Geometry check sheet. Reference: the model listing, model coordinates, mm. Give positions to 0.01 mm unless a question says otherwise; leave off trailing zeros. Write each loop counter-clockwise with the first axis right and the second up, starting at its lowest first coordinate (ties: lowest second). Pieces come first, ordered by that corner, then holes. Notation, with made-up numbers: (-17, -5) - (18, -5) arc R19 cw to (18, 18) - close; hole circle Ø4 at (36, 54). An arc over 180 degrees is marked (long way). Use a Markdown table: item, result.
```python
from build123d import *

# Parameters (mm, degrees)
SKETCH_1_W          = 376.5
SKETCH_1_H          = 280
EXTRUDE_1_DEPTH     = 5
SKETCH_2_R          = 26.25
CUT_EXTRUDE_1_DEPTH = 5
SKETCH_3_R          = 3
EXTRUDE_2_DEPTH     = 5
EXTRUDE_START       = 5
SKETCH_4_R          = 3
EXTRUDE_3_DEPTH     = 5


with BuildPart() as part:
    # 草图1 → 凸台-拉伸1 (new body)
    with BuildSketch(Plane.XY):
        with Locations((188.25, 140)):
            Rectangle(SKETCH_1_W, SKETCH_1_H)
    extrude(amount=EXTRUDE_1_DEPTH)

    # 草图2 → 切除-拉伸1 (cut)
    with BuildSketch(Plane.XY.offset(5)):
        with Locations(Location((84.25, 203.497422612, 0), (0, 0, 180))):
            Circle(SKETCH_2_R)
        with Locations(Location((188.25, 228.989690448, 0), (0, 0, 180))):
            Circle(SKETCH_2_R)
        with Locations(Location((160.25, 180.492267836, 0), (0, 0, 180))):
            Circle(SKETCH_2_R)
        with Locations(Location((216.25, 180.492267836, 0), (0, 0, 180))):
            Circle(SKETCH_2_R)
        with Locations(Location((244.25, 131.994845224, 0), (0, 0, 180))):
            Circle(SKETCH_2_R)
        with Locations(Location((132.25, 131.994845224, 0), (0, 0, 180))):
            Circle(SKETCH_2_R)
        with Locations(Location((188.25, 131.994845224, 0), (0, 0, 180))):
            Circle(SKETCH_2_R)
        with Locations(Location((272.25, 83.497422612, 0), (0, 0, 180))):
            Circle(SKETCH_2_R)
        with Locations(Location((216.25, 83.497422612, 0), (0, 0, 180))):
            Circle(SKETCH_2_R)
        with Locations(Location((104.25, 83.497422612, 0), (0, 0, 180))):
            Circle(SKETCH_2_R)
        with Locations(Location((160.25, 83.497422612, 0), (0, 0, 180))):
            Circle(SKETCH_2_R)
        with Locations(Location((300.25, 35, 0), (0, 0, 180))):
            Circle(SKETCH_2_R)
        with Locations(Location((244.25, 35, 0), (0, 0, 180))):
            Circle(SKETCH_2_R)
        with Locations(Location((188.25, 35, 0), (0, 0, 180))):
            Circle(SKETCH_2_R)
        with Locations(Location((132.25, 35, 0), (0, 0, 180))):
            Circle(SKETCH_2_R)
        with Locations(Location((76.25, 35, 0), (0, 0, 180))):
            Circle(SKETCH_2_R)
    extrude(amount=-CUT_EXTRUDE_1_DEPTH, mode=Mode.SUBTRACT)

    # 草图3 → 凸台-拉伸2 (add)
    with BuildSketch(Plane.ZY):
        with Locations(Location((2.5, 210, 0), (0, 0, 213.557309762))):
            Circle(SKETCH_3_R)
        with Locations(Location((2.5, 95, 0), (0, 0, 213.557309762))):
            Circle(SKETCH_3_R)
    extrude(amount=EXTRUDE_2_DEPTH)

    # 草图4 → 凸台-拉伸3 (add)
    with BuildSketch(Plane(origin=(376.5, 0, 0), x_dir=(0, 0, -1), z_dir=(1, 0, 0)).offset(EXTRUDE_START)):
        with Locations(Location((-2.5, 210, 0), (0, 0, 326.442690238))):
            Circle(SKETCH_4_R)
        with Locations(Location((-2.5, 95, 0), (0, 0, 326.442690238))):
            Circle(SKETCH_4_R)
    extrude(amount=-EXTRUDE_3_DEPTH)


solid = part.part
```
1) Material ranges on L1, parallel to Y at x = 244.25, z = 2.4; L2, parallel to Y at x = 188.25, z = 1.7; L3, parallel to X at y = 129.5, z = 0.9, recorded low to high. Write a range as from..to.
Working result:
| item | result |
|---|---|
| L1 | y = 0..8.75, 61.25..105.74, 158.24..280 |
| L2 | y = 0..8.75, 61.25..105.74, 158.24..202.74, 255.24..280 |
| L3 | x = 0..106.12, 158.38..162.12, 214.38..218.12, 270.38..376.5 |
2) Section check D-D on y = 247.5. Record the boundary of the cut face in (x, z), then the cut area to 3 significant figures.
Working result:
| item | result |
|---|---|
| outline | (0, 0) - (169.64, 0) - (169.64, 5) - (0, 5) - close; (206.86, 0) - (376.5, 0) - (376.5, 5) - (206.86, 5) - close |
| area | 1,700 mm² |
3) Section check B-B on x = 118.5. Record the boundary of the cut face in (y, z).
Working result:
| item | result |
|---|---|
| outline | (0, 0) - (12.64, 0) - (12.64, 5) - (0, 5) - close; (57.36, 0) - (61.45, 0) - (61.45, 5) - (57.36, 5) - close; (105.54, 0) - (109.63, 0) - (109.63, 5) - (105.54, 5) - close; (154.36, 0) - (280, 0) - (280, 5) - (154.36, 5) - close |
4) Depth check by flat-ended pin: P1, Ø1, axis at y = 107.5, z = 4, coming from the -X side; P2, Ø1.5, axis at y = 217.5, z = 2.5, coming from the +X side; P3, Ø2, axis at x = 124, y = 243.5, coming from the +Z side. Enter the tip coordinate at first touch or a pass-through.
Working result:
| item | result |
|---|---|
| P1 | stops at x = 0 |
| P2 | stops at x = 376.5 |
| P3 | stops at z = 5 |
5) Section check C-C on x = 286. Record the boundary of the cut face in (y, z), then the cut area to 3 significant figures.
Working result:
| item | result |
|---|---|
| outline | (0, 0) - (12.95, 0) - (12.95, 5) - (0, 5) - close; (57.05, 0) - (61.14, 0) - (61.14, 5) - (57.05, 5) - close; (105.86, 0) - (280, 0) - (280, 5) - (105.86, 5) - close |
| area | 956 mm² |
6) Mould release check, pull along Y, two halves, no side actions. Record for faces 1 (the flat face through (186, 173, 0)), 2 (the cylindrical face through (298.475, 82.343, 2.535)): pulls with the +Y half, pulls with the -Y half, needs draft (parallel to the pull), parting line crosses it, or undercut.
Working result:
| item | result |
|---|---|
| face 1 | needs draft |
| face 2 | undercut |
7) Section check A-A on y = 41. Record the boundary of the cut face in (x, z).
Working result:
| item | result |
|---|---|
| outline | (0, 0) - (50.69, 0) - (50.69, 5) - (0, 5) - close; (101.81, 0) - (106.69, 0) - (106.69, 5) - (101.81, 5) - close; (157.81, 0) - (162.69, 0) - (162.69, 5) - (157.81, 5) - close; (213.81, 0) - (218.69, 0) - (218.69, 5) - (213.81, 5) - close; (269.81, 0) - (274.69, 0) - (274.69, 5) - (269.81, 5) - close; (325.81, 0) - (376.5, 0) - (376.5, 5) - (325.81, 5) - close |
